Source: CAD feature listing. Evaluate the final solid. Frame: model axes, mm. A direction names the side the tool comes from. Give positions to 0.01 mm unless a question says otherwise; leave off trailing zeros. Write each loop counter-clockwise with the first axis right and the second up, starting at its lowest first coordinate (ties: lowest second). Pieces come first, ordered by that corner, then holes. Notation, with made-up numbers: (89.5, -38.5) -> (107.5, -38.5) arc R26 cw to (107.5, -23.5) -> close; hole circle Ø5 at (84, 7). An arc over 180 degrees is marked (long way). Answer as a JSON object with one key per item and string values. Group by question number.
Item 1: Pull-direction query (X, two-part tool) for faces 3 (the face through (83, 3, -83)), 4 (the face through (-101.6, 3, 33)), 5 (the face through (-1, 3, 101.6)), 6 (the face through (16, 3, 10.832)); classes: pulls with the +X half, pulls with the -X half, needs draft (parallel to the pull), parting line crosses it, or undercut.
Item 2: Section query C-C on y = 3.25. Give the number of separate pieces and of enclosed holes in the cut face, plus the area to 3 significant figures.
Item 3: First-contact query: pin 1 Ø4 at (x, z) = (28.52, 60.97) entering from -Y; pin 2 Ø1 at (x, y) = (-68, 1.5) entering from -Z. Flat tips, straight axial feed; report the tip coordinate or a pass-through.
Item 4: Section query B-B on x = -73.66. Return the cut outline in (y, z).
Item 5: Section query D-D on z = -72. Return the cut outline in (x, y), plus the area to 3 significant figures.
Item 6: Section query A-A on z = 26.5. Return the cut outline in (x, y), plus the area to 3 significant figures.
Item 7: Access query for faces 1 (the face through (-1, 3, -101.6)), 2 (the face through (-13.112, 3, 42)). Directions: +Z, -Z, +X, -X, +Y, -Y. A direction counts if a zero-diameter tool reaches every point of the face in a straight line with its end or side. Return the directions, or none.
Item 8: Ray query, probe 1 along X at (y, z) = (3.25, 46.5); probe 2 along X at (y, z) = (3.5, -13); probe 3 along Z at (x, y) = (15, 1). Return the intervals inside material, ascending. Write a range as from..to.
from build123d import *

# Parameters (mm, degrees)
SKETCH1_W           = 203.2
SKETCH1_H           = 203.2
BOSS_EXTRUDE1_DEPTH = 6.35
CUT_EXTRUDE1_DEPTH  = 7.35
SKETCH10_R          = 3.175
SKETCH10_W          = 6.35
SKETCH10_H          = 62.924217451
CUT_EXTRUDE4_DEPTH  = 7.35


with BuildPart() as part:
    # Sketch1 → Boss-Extrude1 (new body)
    with BuildSketch(Plane(origin=(0, 0, 0), x_dir=(1, 0, 0), z_dir=(0, 1, 0))):
        Rectangle(SKETCH1_W, SKETCH1_H)
    extrude(amount=BOSS_EXTRUDE1_DEPTH)

    # Sketch2 → Cut-Extrude1 (cut, through all)
    with BuildSketch(Plane(origin=(0, 6.35, 0), x_dir=(1, 0, 0), z_dir=(0, 1, 0))):
        with BuildLine():
            Line((101.6, 38.1), (101.6, 101.6))
            Line((101.6, 101.6), (38.1, 101.6))
            ThreePointArc((38.1, 101.6), (83.001280605, 83.001280605), (101.6, 38.1))
        make_face()
        with BuildLine():
            Line((-38.1, 101.6), (-101.6, 101.6))
            Line((-101.6, 101.6), (-101.6, 38.1))
            ThreePointArc((-101.6, 38.1), (-83.001280605, 83.001280605), (-38.1, 101.6))
        make_face()
    extrude(amount=-CUT_EXTRUDE1_DEPTH, mode=Mode.SUBTRACT)

    # Sketch10 → Cut-Extrude4 (cut, through all)
    with BuildSketch(Plane.XZ):
        with Locations((25.309743879, -12.40083867)):
            Circle(SKETCH10_R)
        with Locations((-25.490256121, -12.40083867)):
            Circle(SKETCH10_R)
        with Locations((-25.490256121, -57.61283867)):
            Circle(SKETCH10_R)
        with Locations((25.309743879, -57.61283867)):
            Circle(SKETCH10_R)
        with Locations((-73.66, 16.002)):
            Circle(SKETCH10_R)
        with Locations((-73.66, 60.965705209)):
            Circle(SKETCH10_R)
        with Locations((-28.696294791, 60.965705209)):
            Circle(SKETCH10_R)
        with Locations((-28.696294791, 16.002)):
            Circle(SKETCH10_R)
        with Locations((28.515782549, 60.965705209)):
            Circle(SKETCH10_R)
        with Locations((73.479487758, 60.965705209)):
            Circle(SKETCH10_R)
        with Locations((73.479487758, 16.002)):
            Circle(SKETCH10_R)
        with Locations((28.515782549, 16.002)):
            Circle(SKETCH10_R)
        with Locations((-16.28703867, 42.293852605)):
            Rectangle(SKETCH10_W, SKETCH10_H)
        with Locations((16.106526428, 42.293852605)):
            Rectangle(SKETCH10_W, SKETCH10_H)
    extrude(amount=-CUT_EXTRUDE4_DEPTH, mode=Mode.SUBTRACT)


solid = part.part
Worked answers:
{
 "1": {"face 3": "pulls with the +X half", "face 4": "pulls with the -X half", "face 5": "needs draft", "face 6": "undercut"},
 "2": {"separate pieces": "1", "enclosed holes": "14", "area": "38,400 mm^2"},
 "3": {"pin 1": "through", "pin 2": "z = -94.38"},
 "4": {"outline": "(0, -90.71) -> (6.35, -90.71) -> (6.35, 12.83) -> (0, 12.83) -> close; (0, 19.18) -> (6.35, 19.18) -> (6.35, 57.79) -> (0, 57.79) -> close; (0, 64.14) -> (6.35, 64.14) -> (6.35, 101.6) -> (0, 101.6) -> close"},
 "5": {"outline": "(-91.79, 0) -> (91.79, 0) -> (91.79, 6.35) -> (-91.79, 6.35) -> close", "area": "1,170 mm^2"},
 "6": {"outline": "(-101.6, 0) -> (-19.46, 0) -> (-19.46, 6.35) -> (-101.6, 6.35) -> close; (-13.11, 0) -> (12.93, 0) -> (12.93, 6.35) -> (-13.11, 6.35) -> close; (19.28, 0) -> (101.6, 0) -> (101.6, 6.35) -> (19.28, 6.35) -> close", "area": "1,210 mm^2"},
 "7": {"face 1": "-Z, +X, -X, +Y, -Y", "face 2": "+Y, -Y"},
 "8": {"probe 1": "-101.6..-19.46, -13.11..12.93, 19.28..101.6", "probe 2": "-101.6..-28.61, -22.37..22.19, 28.43..101.6", "probe 3": "-101.6..10.83, 73.76..101.6"}
}
